```python
from build123d import *

# Parameters (mm, degrees)
BOSS_EXTRUDE1_DEPTH = 100


with BuildPart() as part:
    # Sketch1 → Boss-Extrude1 (new body)
    with BuildSketch(Plane.XY):
        Polygon((18.475208614, 0), (9.237604307, 16), (-9.237604307, 16), (-18.475208614, 0), (-9.237604307, -16), (9.237604307, -16), align=None)
    extrude(amount=BOSS_EXTRUDE1_DEPTH)

    # Sketch2 → Cut-Revolve1 (revolve, cut)
    with BuildSketch(Plane(origin=(0, 0, 0), x_dir=(0, 0, -1), z_dir=(1, 0, 0))):
        Polygon((-100, 16), (-100, 22.884653205), (-96.025143619, 22.884653205), align=None)
        Polygon((0, 22.884653205), (-3.974856381, 22.884653205), (0, 16), align=None)
    revolve(axis=Axis((0, 0, 0), (0, 0, 1)), mode=Mode.SUBTRACT)


solid = part.part
```
Model file for the job. Use its own axes, mm. Round coordinates to 2 decimals unless told otherwise and drop trailing zeros. Write each loop counter-clockwise with the first axis right and the second up, starting at its lowest first coordinate (ties: lowest second). Pieces come first, ordered by that corner, then holes. Notation, with made-up numbers: (-27.5, 9.5) - (-20.5, 9.5) arc R16 cw to (-20.5, 24.5) - close; hole circle Ø5 at (4, 35). An arc over 180 degrees is marked (long way). One line per item, written item: value.
(1) Cut at A-A, the plane z = 76.5. Give the cut face in (x, y), plus the area to 3 significant figures.
Values follow:
outline: (-18.48, 0) - (-9.24, -16) - (9.24, -16) - (18.48, 0) - (9.24, 16) - (-9.24, 16) - close
area: 887 mm²
(2) Drop flat-ended pins along their axis: P1, Ø1, axis at y = 1.5, z = 46.5, coming from the +X side; P2, Ø10, axis at y = 12.5, z = 42, coming from the +X side; P3, Ø1, axis at y = -2, z = 89, coming from the -X side. Give the stop position or say it passes through.
Values follow:
P1: stops at x = 17.9
P2: stops at x = 14.15
P3: stops at x = -17.61
(3) Wall check: probe 1 along Y at (x, z) = (-11.5, 61.5); probe 2 along Y at (x, z) = (-14, 83); probe 3 along X at (y, z) = (-4.5, 54). Give the ranges that are in metal, low to high.
Values follow:
probe 1: y = -12.08 to 12.08
probe 2: y = -7.75 to 7.75
probe 3: x = -15.88 to 15.88
